```python
from build123d import *

# Parameters (mm, degrees)
SKETCH1_R           = 1.5
BOSS_EXTRUDE1_DEPTH = 6


with BuildPart() as part:
    # Sketch1 → Boss-Extrude1 (new body)
    with BuildSketch(Plane(origin=(0, 0, 0), x_dir=(1, 0, 0), z_dir=(0, 1, 0))):
        with BuildLine():
            Line((2.54, 0), (147.46, 0))
            ThreePointArc((147.46, 0), (149.256051224, 0.743948776), (150, 2.54))
            Line((150, 2.54), (150, 177.46))
            ThreePointArc((150, 177.46), (149.256051224, 179.256051224), (147.46, 180))
            Line((147.46, 180), (2.54, 180))
            ThreePointArc((2.54, 180), (0.743948776, 179.256051224), (0, 177.46))
            Line((0, 177.46), (0, 2.54))
            ThreePointArc((0, 2.54), (0.743948776, 0.743948776), (2.54, 0))
        make_face()
        with Locations((33.500605467, 5)):
            Circle(SKETCH1_R, mode=Mode.SUBTRACT)
        with Locations((8.500605467, 5)):
            Circle(SKETCH1_R, mode=Mode.SUBTRACT)
        with Locations((141.499394533, 5)):
            Circle(SKETCH1_R, mode=Mode.SUBTRACT)
        with Locations((116.499394533, 5)):
            Circle(SKETCH1_R, mode=Mode.SUBTRACT)
        with Locations((75, 155.5)):
            Circle(SKETCH1_R, mode=Mode.SUBTRACT)
        with Locations((39, 155.5)):
            Circle(SKETCH1_R, mode=Mode.SUBTRACT)
        with Locations((21, 155.5)):
            Circle(SKETCH1_R, mode=Mode.SUBTRACT)
        with Locations((57, 155.5)):
            Circle(SKETCH1_R, mode=Mode.SUBTRACT)
        with Locations((93, 155.5)):
            Circle(SKETCH1_R, mode=Mode.SUBTRACT)
        with Locations((111, 155.5)):
            Circle(SKETCH1_R, mode=Mode.SUBTRACT)
        with Locations((129, 155.5)):
            Circle(SKETCH1_R, mode=Mode.SUBTRACT)
        with Locations((129, 175.5)):
            Circle(SKETCH1_R, mode=Mode.SUBTRACT)
        with Locations((111, 175.5)):
            Circle(SKETCH1_R, mode=Mode.SUBTRACT)
        with Locations((93, 175.5)):
            Circle(SKETCH1_R, mode=Mode.SUBTRACT)
        with Locations((75, 175.5)):
            Circle(SKETCH1_R, mode=Mode.SUBTRACT)
        with Locations((57, 175.5)):
            Circle(SKETCH1_R, mode=Mode.SUBTRACT)
        with Locations((39, 175.5)):
            Circle(SKETCH1_R, mode=Mode.SUBTRACT)
        with Locations((21, 175.5)):
            Circle(SKETCH1_R, mode=Mode.SUBTRACT)
        with Locations((145, 100)):
            Circle(SKETCH1_R, mode=Mode.SUBTRACT)
        with Locations((95, 142)):
            Circle(SKETCH1_R, mode=Mode.SUBTRACT)
        with Locations((145, 90)):
            Circle(SKETCH1_R, mode=Mode.SUBTRACT)
        with Locations((5, 90)):
            Circle(SKETCH1_R, mode=Mode.SUBTRACT)
        with Locations((75, 80)):
            Circle(SKETCH1_R, mode=Mode.SUBTRACT)
        with Locations((75, 40)):
            Circle(SKETCH1_R, mode=Mode.SUBTRACT)
        with BuildLine():
            Line((133.5, 167.5), (124.5, 167.5))
            ThreePointArc((124.5, 167.5), (122.5, 165.5), (124.5, 163.5))
            Line((124.5, 163.5), (133.5, 163.5))
            ThreePointArc((133.5, 163.5), (135.5, 165.5), (133.5, 167.5))
        make_face(mode=Mode.SUBTRACT)
        with BuildLine():
            Line((16.5, 167.5), (25.5, 167.5))
            ThreePointArc((25.5, 167.5), (27.5, 165.5), (25.5, 163.5))
            Line((25.5, 163.5), (16.5, 163.5))
            ThreePointArc((16.5, 163.5), (14.5, 165.5), (16.5, 167.5))
        make_face(mode=Mode.SUBTRACT)
        with BuildLine():
            Line((34.5, 167.5), (43.5, 167.5))
            ThreePointArc((43.5, 167.5), (45.5, 165.5), (43.5, 163.5))
            Line((43.5, 163.5), (34.5, 163.5))
            ThreePointArc((34.5, 163.5), (32.5, 165.5), (34.5, 167.5))
        make_face(mode=Mode.SUBTRACT)
        with BuildLine():
            Line((52.5, 167.5), (61.5, 167.5))
            ThreePointArc((61.5, 167.5), (63.5, 165.5), (61.5, 163.5))
            Line((61.5, 163.5), (52.5, 163.5))
            ThreePointArc((52.5, 163.5), (50.5, 165.5), (52.5, 167.5))
        make_face(mode=Mode.SUBTRACT)
        with BuildLine():
            Line((70.5, 167.5), (79.5, 167.5))
            ThreePointArc((79.5, 167.5), (81.5, 165.5), (79.5, 163.5))
            Line((79.5, 163.5), (70.5, 163.5))
            ThreePointArc((70.5, 163.5), (68.5, 165.5), (70.5, 167.5))
        make_face(mode=Mode.SUBTRACT)
        with BuildLine():
            Line((115.5, 167.5), (106.5, 167.5))
            ThreePointArc((106.5, 167.5), (104.5, 165.5), (106.5, 163.5))
            Line((106.5, 163.5), (115.5, 163.5))
            ThreePointArc((115.5, 163.5), (117.5, 165.5), (115.5, 167.5))
        make_face(mode=Mode.SUBTRACT)
        with BuildLine():
            Line((97.5, 167.5), (88.5, 167.5))
            ThreePointArc((88.5, 167.5), (86.5, 165.5), (88.5, 163.5))
            Line((88.5, 163.5), (97.5, 163.5))
            ThreePointArc((97.5, 163.5), (99.5, 165.5), (97.5, 167.5))
        make_face(mode=Mode.SUBTRACT)
        with BuildLine():
            Line((10.000605467, 30), (10.000605467, 27))
            ThreePointArc((10.000605467, 27), (8.500605467, 25.5), (7.000605467, 27))
            Line((7.000605467, 27), (7.000605467, 30))
            ThreePointArc((7.000605467, 30), (8.500605467, 31.5), (10.000605467, 30))
        make_face(mode=Mode.SUBTRACT)
        with BuildLine():
            Line((35.000605467, 30), (35.000605467, 27))
            ThreePointArc((35.000605467, 27), (33.500605467, 25.5), (32.000605467, 27))
            Line((32.000605467, 27), (32.000605467, 30))
            ThreePointArc((32.000605467, 30), (33.500605467, 31.5), (35.000605467, 30))
        make_face(mode=Mode.SUBTRACT)
        with BuildLine():
            Line((114.999394533, 30), (114.999394533, 27))
            ThreePointArc((114.999394533, 27), (116.499394533, 25.5), (117.999394533, 27))
            Line((117.999394533, 27), (117.999394533, 30))
            ThreePointArc((117.999394533, 30), (116.499394533, 31.5), (114.999394533, 30))
        make_face(mode=Mode.SUBTRACT)
        with BuildLine():
            Line((139.999394533, 30), (139.999394533, 27))
            ThreePointArc((139.999394533, 27), (141.499394533, 25.5), (142.999394533, 27))
            Line((142.999394533, 27), (142.999394533, 30))
            ThreePointArc((142.999394533, 30), (141.499394533, 31.5), (139.999394533, 30))
        make_face(mode=Mode.SUBTRACT)
    extrude(amount=BOSS_EXTRUDE1_DEPTH)


solid = part.part
```
Geometry check sheet. Reference: the model listing, model coordinates, mm. A direction names the side the tool comes from. Give positions to 0.01 mm unless a question says otherwise; leave off trailing zeros. Write item = value, one per line. Start each with the question number.
1) Scan lines: L1, parallel to Z at x = 111, y = 0.5; L2, parallel to X at y = 3.55, z = -5; L3, parallel to Z at x = 59.5, y = 4. Record each from-to range of solid material in increasing order.
2) Draft check along X on faces 3 (the flat face through (57, 3, -167.5)), 4 (the flat face through (74, 6, -91)). Enter one of: released by +X, released by -X, zero draft, split by the parting line, or undercut.
3) Section check A-A (y = 5.05). Count the separate pieces of the cut face and the enclosed holes in it, then the cut area to 3 significant figures.
4) Access from +Z, -Z, +X, -X, +Y, -Y to the whole of each face (thin tool, end or side, straight path). Record for faces 1 (the flat face through (76, 3, -180)), 2 (the flat face through (129, 3, -167.5)).
Geometry check:
q1.L1 = -180 to -177, -174 to -167.5, -163.5 to -157, -154 to 0
q1.L2 = 0 to 7, 10 to 32, 35 to 115, 118 to 140, 143 to 150
q1.L3 = -180 to -167.5, -163.5 to 0
q2.face_3 = undercut
q2.face_4 = zero draft
q3.separate_pieces = 1
q3.enclosed_holes = 35
q3.area = 26,400 mm2
q4.face_1 = -Z, +X, -X, +Y, -Y
q4.face_2 = +Y, -Y
